Part model, mm, in its own coordinate system. Round coordinates to 2 decimals unless told otherwise and drop trailing zeros. Write each loop counter-clockwise with the first axis right and the second up, starting at its lowest first coordinate (ties: lowest second). Pieces come first, ordered by that corner, then holes. Notation, with made-up numbers: M 44.5,7 L 99.5,7 A14 ccw 99.5,34 Z; hole C 75.25,62 d11. An arc over 180 degrees is marked long. Use one line per item in the form item = value. Start each with the question number.
Item 1: Cut at B-B, the plane y = -0.15. Give the cut face in (x, z) (3 decimals).
Item 2: Cut at A-A, the plane z = 5.5. Give the cut face in (x, y) (3 decimals).
Item 3: Probe L1, parallel to Z at x = 4.7, y = -0.05; L2, parallel to X at y = 0.1, z = 7.5 (3 decimals); L3, parallel to X at y = -0.1, z = -2.75. List the from-to ranges inside material, lowest first.
Item 4: Cut at D-D, the plane z = -0.25. Give the cut face in (x, y) (3 decimals), then the cut area to 3 significant figures.
Item 5: Cut at C-C, the plane x = 4.55. Give the cut face in (y, z) (3 decimals).
from build123d import *

# Parameters (mm, degrees)
BOX066_W                = 2.9
BOX066_H                = 0.55
BOX066_DEPTH            = 15
BOX067_W                = 1.25
BOX067_H                = 0.55
BOX067_DEPTH            = 6
BOX068_W                = 1.1
BOX068_H                = 0.6
BOX068_DEPTH            = 2
BOX070_W                = 1
BOX070_H                = 0.55
BOX070_DEPTH            = 6
BOX069_W                = 3
BOX069_H                = 0.55
BOX069_DEPTH            = 4
CHAMFER030_SIZE2        = 0.65
CHAMFER030_SIZE         = 2
CHAMFER031_ANGLE        = 33
CHAMFER031_SIZE         = 0.5
CHAMFER033_ANGLE        = 56
CHAMFER033_SIZE         = 0.33
CHAMFER032_ANGLE        = 26.565
CHAMFER032_SIZE         = 1.98
BODY028_PLACEMENT_ANGLE = 180


with BuildPart() as part:
    # Box066 → Box066 (join)
    with BuildSketch(Plane(origin=(-4.95, -0.275, 0), x_dir=(1, 0, 0), z_dir=(0, 0, 1))):
        with Locations((1.45, 0.275)):
            Rectangle(BOX066_W, BOX066_H)
    extrude(amount=BOX066_DEPTH)

    # Box067 → Box067 (cut)
    with BuildSketch(Plane(origin=(-4.125, -0.275, 9), x_dir=(1, 0, 0), z_dir=(0, 0, 1))):
        with Locations((0.625, 0.275)):
            Rectangle(BOX067_W, BOX067_H)
    extrude(amount=BOX067_DEPTH, mode=Mode.SUBTRACT)

    # Box068 → Box068 (cut)
    with BuildSketch(Plane(origin=(-3, -0.3, 13), x_dir=(1, 0, 0), z_dir=(0, 0, 1))):
        with Locations((0.55, 0.3)):
            Rectangle(BOX068_W, BOX068_H)
    extrude(amount=BOX068_DEPTH, mode=Mode.SUBTRACT)

    # Box070 → Box070 (join)
    with BuildSketch(Plane(origin=(-5.95, -0.275, 0), x_dir=(1, 0, 0), z_dir=(0, 0, 1))):
        with Locations((0.5, 0.275)):
            Rectangle(BOX070_W, BOX070_H)
    extrude(amount=BOX070_DEPTH)

    # Box069 → Box069 (cut)
    with BuildSketch(Plane(origin=(-4.95, 0.275, 4), x_dir=(1, 0, 0), z_dir=(0, 0, -1))):
        with Locations((1.5, 0.275)):
            Rectangle(BOX069_W, BOX069_H)
    extrude(amount=BOX069_DEPTH, mode=Mode.SUBTRACT)

    # Chamfer030
    chamfer030_edges = [part.edges().sort_by_distance(p)[0] for p in [
        (-2.05, 0, 4),
    ]]
    chamfer030_side = part.faces().sort_by_distance((-2.05, 0, 8.5))[0]
    chamfer(chamfer030_edges, length=CHAMFER030_SIZE, length2=CHAMFER030_SIZE2, reference=chamfer030_side)

    # Chamfer031
    chamfer031_edges = [part.edges().sort_by_distance(p)[0] for p in [
        (-4.95, 0, 0),
    ]]
    chamfer031_side = part.faces().sort_by_distance((-4.95, 0, 2))[0]
    chamfer(chamfer031_edges, length=CHAMFER031_SIZE, angle=CHAMFER031_ANGLE, reference=chamfer031_side)

    # Chamfer033
    chamfer033_edges = [part.edges().sort_by_distance(p)[0] for p in [
        (-5.95, 0, 0),
    ]]
    chamfer033_side = part.faces().sort_by_distance((-5.612352, 0, 0))[0]
    chamfer(chamfer033_edges, length=CHAMFER033_SIZE, angle=CHAMFER033_ANGLE, reference=chamfer033_side)

    # Chamfer032
    chamfer032_edges = [part.edges().sort_by_distance(p)[0] for p in [
        (-5.95, 0, 6),
    ]]
    chamfer032_side = part.faces().sort_by_distance((-5.95, 0, 3.244623))[0]
    chamfer(chamfer032_edges, length=CHAMFER032_SIZE, angle=CHAMFER032_ANGLE, reference=chamfer032_side)


with BuildPart() as part_1:
    # Body028 placement: moved
    add(part.part.moved(Location((0, 0, -4))).rotate(Axis((0, 0, -4), (0, 0, 1)), BODY028_PLACEMENT_ANGLE))


solid = part_1.part
Model answer:
q1.outline = M 2.05,2 L 2.7,0 L 4.95,0 L 4.95,-3.5 L 5.275,-4 L 5.62,-4 L 5.95,-3.511 L 5.95,0.02 L 4.96,2 L 4.95,2 L 4.95,11 L 4.125,11 L 4.125,5 L 2.875,5 L 2.875,9 L 2.05,9 Z
q2.outline = M 2.05,-0.275 L 2.875,-0.275 L 2.875,0.275 L 2.05,0.275 Z; M 4.125,-0.275 L 4.95,-0.275 L 4.95,0.275 L 4.125,0.275 Z
q3.L1 = 0 to 11
q3.L2 = 2.05 to 2.875, 4.125 to 4.95
q3.L3 = 4.95 to 5.95
q4.outline = M 4.95,-0.275 L 5.95,-0.275 L 5.95,0.275 L 4.95,0.275 Z
q4.area = 0.550 mm²
q5.outline = M -0.275,0 L 0.275,0 L 0.275,11 L -0.275,11 Z
